from build123d import *

# Parameters (mm, degrees)
F1_DEPTH = 63.5
F0_W     = 25.4
F0_H     = 19.05
F2_DEPTH = 25.4
F3_DEPTH = 7.9375
F5_R     = 6.35


with BuildPart() as f1:
    # F0 (on Front) → F1 (new body, symmetric)
    with BuildSketch(Plane.XZ):
        Polygon((41.275, -9.525), (41.275, 9.525), (22.225, 9.525), (-41.275, 9.525), (-41.275, -9.525), align=None)
    extrude(amount=F1_DEPTH, both=True)

    # F0 (on Front) → F2 (join, symmetric)
    with BuildSketch(Plane.XZ):
        with BuildLine():
            Line((22.225, 9.525), (41.275, 9.525))
            Line((41.275, 9.525), (41.275, 27.0002))
            ThreePointArc((41.275, 27.0002), (45.92468, 38.22552), (57.15, 42.8752))
            Line((57.15, 42.8752), (60.325, 42.8752))
            Line((60.325, 42.8752), (60.325, 61.9252))
            add(Edge.make_bspline(
                [(51.823545, 61.516638), (54.671503, 61.742605), (57.509493, 61.880867), (60.325, 61.9252)],
                knots=[107.525137, 107.525137, 107.525137, 107.525137, 114.316845, 114.316845, 114.316845, 114.316845], degree=3))
            ThreePointArc((51.823545, 61.516638), (30.637908, 49.734856), (22.225, 27.0002))
            Line((22.225, 27.0002), (22.225, 9.525))
        make_face()
        with Locations((73.025, 52.4002)):
            Rectangle(F0_W, F0_H)
    extrude(amount=F2_DEPTH, both=True)

    # F0 (on Front) → F3 (join, symmetric)
    with BuildSketch(Plane.XZ):
        with BuildLine():
            Line((-41.275, 9.525), (22.225, 9.525))
            Line((22.225, 9.525), (22.225, 27.0002))
            ThreePointArc((22.225, 27.0002), (30.637908, 49.734856), (51.823545, 61.516638))
            add(Edge.make_bspline(
                [(-41.275, 9.525), (-40.851534, 32.378485), (6.735176, 57.939164), (51.823545, 61.516638)],
                knots=[0, 0, 0, 0, 107.525137, 107.525137, 107.525137, 107.525137], degree=3))
        make_face()
    extrude(amount=F3_DEPTH, both=True)

    # F0 (on Front) → F4 (revolve)
    with BuildSketch(Plane.XZ):
        Polygon((85.725, 61.9252), (85.725, 42.8752), (85.725, 38.1), (111.125, 38.1), (111.125, 66.675), (85.725, 66.675), align=None)
    revolve(axis=Axis((85.725, 0, 52.3875), (0, 0, 1)))

    # F5
    f5_edges = [f1.edges().sort_by_distance(p)[0] for p in [
        (41.275, -63.5, 0),
        (-41.275, -63.5, 0),
        (41.275, 63.5, 0),
        (-41.275, 63.5, 0),
    ]]
    fillet(f5_edges, radius=F5_R)


solid = f1.part
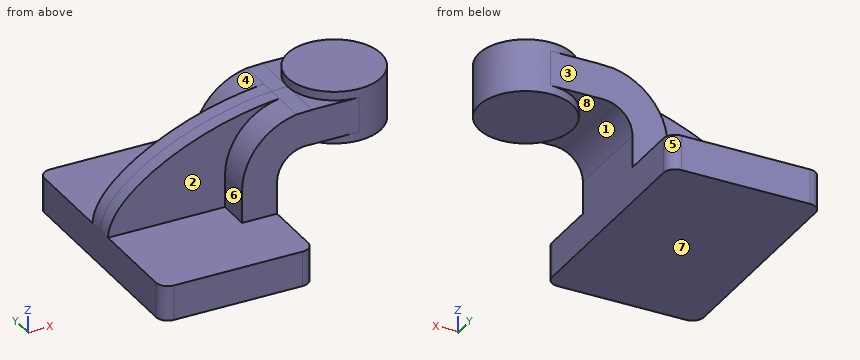
Geometry check sheet. Reference: the model listing, model coordinates, mm. Face numbers are marked on the shaded views. A direction names the side the tool comes from. Round coordinates to 2 decimals unless told otherwise and drop trailing zeros. Order: outer loops, then holes, each group sorted by start corner. A loop starts at its lowest first (then second) coordinate and runs counter-clockwise, first axis right, second up. Notation, with made-up numbers: M 73.5,4.25 L 99.5,4.25 A20 cw 99.5,26.25 Z; hole C 12,14 d9. An arc over 180 degrees is marked long. Answer in a Markdown table with one row per item.
(1) Sectioned sample at C-C, the plane y = 30.5. Record the cut outline in (x, z) (3 decimals), and give its area (3 significant figures).
Responses:
| item | result |
|---|---|
| outline | M -41.275,-9.525 L 41.275,-9.525 L 41.275,9.525 L -41.275,9.525 Z |
| area | 1,570 mm² |
(2) Tool access check on the marked faces 1, 2, 3 and 4. Record the directions out of +Z, -Z, +X, -X, +Y, -Y that give a thin tool (end or side, any length) a straight path to the whole face; none if there is none.
Responses:
| item | result |
|---|---|
| face 1 | -Z, +Y, -Y |
| face 2 | +Z, -X, -Y |
| face 3 | +Z, +X, -X, +Y |
| face 4 | +Z, -X, +Y |
(3) Sectioned sample at B-B, the plane x = 69. Record the cut outline in (y, z) (3 decimals), and give its area (3 significant figures).
Responses:
| item | result |
|---|---|
| outline | M -25.4,42.875 L -19.116,42.875 L -19.116,38.1 L 19.116,38.1 L 19.116,42.875 L 25.4,42.875 L 25.4,61.925 L 19.116,61.925 L 19.116,66.675 L -19.116,66.675 L -19.116,61.925 L -25.4,61.925 Z |
| area | 1,330 mm² |
(4) Go/stop test with flat-tipped pins: P1, Ø8, axis at x = 50, y = -19, coming from the +Z side; P2, Ø5, axis at x = 61, y = -25.5, coming from the +Z side; P3, Ø8.5, axis at x = 74.5, y = -11.5, coming from the -Z side; P4, Ø6, axis at x = 8.5, z = 10.5, coming from the -Y side. Record where each tip stops, or that it passes through.
Responses:
| item | result |
|---|---|
| P1 | stops at z = 61.67 |
| P2 | stops at z = 61.93 |
| P3 | stops at z = 38.1 |
| P4 | stops at y = -63.5 |
(5) Sectioned sample at A-A, the plane z = -3. Record the cut outline in (x, y) (3 decimals), and give its area (3 significant figures).
Responses:
| item | result |
|---|---|
| outline | M -41.275,-57.15 A6.35 ccw -34.925,-63.5 L 34.925,-63.5 A6.35 ccw 41.275,-57.15 L 41.275,57.15 A6.35 ccw 34.925,63.5 L -34.925,63.5 A6.35 ccw -41.275,57.15 Z |
| area | 10,400 mm² |
(6) Draft check along X on the marked faces 5, 6, 7 and 8. Enter one of: released by +X, released by -X, zero draft, split by the parting line, or undercut.
Responses:
| item | result |
|---|---|
| face 5 | released by +X |
| face 6 | released by -X |
| face 7 | zero draft |
| face 8 | undercut |
(7) Scan lines: probe 1 along Z at (x, y) = (20, -14) (3 decimals); probe 2 along X at (y, z) = (35.5, 4) (3 decimals); probe 3 along Y at (x, z) = (-17.5, 36). Record each from-to range of solid material in increasing order. Write a range as from..to.
Responses:
| item | result |
|---|---|
| probe 1 | z = -9.525..9.525 |
| probe 2 | x = -41.275..41.275 |
| probe 3 | y = -7.94..7.94 |
